The model under review builds one solid part; all positions refer to its coordinate system, in mm. A direction names the side the tool comes from. Coordinates: 2 decimals unless noted, no trailing zeros. Write each loop counter-clockwise with the first axis right and the second up, starting at its lowest first coordinate (ties: lowest second). Pieces come first, ordered by that corner, then holes.
```python
from build123d import *

# Parameters (mm, degrees)
SKETCH2_R           = 1.3
CUT_EXTRUDE1_DEPTH  = 7
SKETCH4_R           = 4.75
CUT_EXTRUDE2_DEPTH  = 82.929848041
FILLET1_R           = 15
FILLET2_R           = 4
SKETCH5_R           = 7
BOSS_EXTRUDE1_DEPTH = 5
CHAMFER1_SIZE       = 1


with BuildPart() as part:
    # Sketch1 → Revolve1 (revolve)
    with BuildSketch(Plane.XY, mode=Mode.PRIVATE) as revolve1_sk:
        Polygon((0, -40), (0, 40), (-12.5, 40), (-12.5, 37), (-8, 28), (-8, -28), (-12.5, -37), (-12.5, -40), align=None)
    revolve(revolve1_sk.sketch.rotate(Axis((0, -40, 0), (0, 1, 0)), 270), axis=Axis((0, -40, 0), (0, 1, 0)))

    # Sketch2 → Cut-Extrude1 (cut)
    with BuildSketch(Plane(origin=(0, 40, 0), x_dir=(1, 0, 0), z_dir=(0, 1, 0))):
        with Locations(Location((-6, 6, 0), (0, 0, 270))):
            Circle(SKETCH2_R)
        with Locations(Location((6, 6, 0), (0, 0, 270))):
            Circle(SKETCH2_R)
        with Locations(Location((-6, -6, 0), (0, 0, 270))):
            Circle(SKETCH2_R)
        with Locations(Location((6, -6, 0), (0, 0, 270))):
            Circle(SKETCH2_R)
    cut_extrude1 = extrude(amount=-CUT_EXTRUDE1_DEPTH, mode=Mode.SUBTRACT)

    # Mirror1: Cut-Extrude1 across plane
    add(cut_extrude1.mirror(Plane.ZX), mode=Mode.SUBTRACT)

    # Sketch3 → Cut-Revolve1 (revolve, cut)
    with BuildSketch(Plane(origin=(0, 0, 0), x_dir=(0, 0, -1), z_dir=(1, 0, 0))):
        Polygon((-5, 31.7), (0, 36.7), (0, -36.7), (-5, -31.7), align=None)
    revolve(axis=Axis((0, 36.7, 0), (0, -1, 0)), mode=Mode.SUBTRACT)

    # Sketch4 → Cut-Extrude2 (cut, through all)
    with BuildSketch(Plane(origin=(0, 40, 0), x_dir=(1, 0, 0), z_dir=(0, 1, 0))):
        with Locations(Location((0, 0, 0), (0, 0, 270))):
            Circle(SKETCH4_R)
    extrude(amount=-CUT_EXTRUDE2_DEPTH, mode=Mode.SUBTRACT)

    # Fillet1
    fillet1_edges = [part.edges().sort_by_distance(p)[0] for p in [
        (0, -28, 8),
        (0, 28, 8),
    ]]
    fillet(fillet1_edges, radius=FILLET1_R)

    # Fillet2
    # the kernel refuses this fillet: 4 mm, written as the material it adds along each edge
    with BuildSketch(Plane(origin=(0, 31.7, 0), x_dir=(0, 0, 1), z_dir=(1, 0, 0))) as fillet2_piece_1:
        with BuildLine():
            CenterArc((1, 1.141941091), FILLET2_R, 339.635865194, 20.364134806)
            Line((5, 1.141941091), (5.08, 1.141941091))
            Line((5.08, 1.141941091), (5.08, 0))
            Line((5.08, 0), (5.056568542, -0.056568542))
            ThreePointArc((5.056568542, -0.056568542), (4.931568542, -0.181568542), (4.825, -0.277838822))
            Line((4.825, -0.277838822), (4.75, -0.25))
        make_face()
    revolve(axis=Axis((0, 31.7, 0), (0, -1, 0)))
    with BuildSketch(Plane(origin=(0, -31.7, 0), x_dir=(0, 0, 1), z_dir=(1, 0, 0))) as fillet2_piece_2:
        with BuildLine():
            CenterArc((1, -1.141941091), FILLET2_R, 0, 20.364134806)
            Line((4.75, 0.25), (4.825, 0.277838822))
            ThreePointArc((4.825, 0.277838822), (4.931568542, 0.181568542), (5.056568542, 0.056568542))
            Line((5.056568542, 0.056568542), (5.08, 0))
            Line((5.08, 0), (5.08, -1.141941091))
            Line((5.08, -1.141941091), (5, -1.141941091))
        make_face()
    revolve(axis=Axis((0, -31.7, 0), (0, -1, 0)))

    # Sketch5 → Boss-Extrude1 (add, symmetric)
    with BuildSketch(Plane(origin=(0, 0, 0), x_dir=(1, 0, 0), z_dir=(0, 1, 0))):
        Polygon((4.618802154, 8), (-4.618802154, 8), (-9.237604307, 0), (-4.618802154, -8), (4.618802154, -8), (9.237604307, 0), align=None)
        Circle(SKETCH5_R, mode=Mode.SUBTRACT)
    extrude(amount=BOSS_EXTRUDE1_DEPTH, both=True)

    # Sketch6 → Cut-Revolve2 (revolve, cut)
    with BuildSketch(Plane.XY, mode=Mode.PRIVATE) as cut_revolve2_sk:
        Polygon((-8, 5), (-9.237604307, 3.762395693), (-9.237604307, 5), align=None)
    cut_revolve2 = revolve(cut_revolve2_sk.sketch.rotate(Axis((0, -40, 0), (0, -1, 0)), 270), axis=Axis((0, -40, 0), (0, -1, 0)), mode=Mode.SUBTRACT)

    # Mirror2: Cut-Revolve2 across plane
    add(cut_revolve2.mirror(Plane.ZX), mode=Mode.SUBTRACT)

    # Chamfer1
    chamfer1_edges = [part.edges().sort_by_distance(p)[0] for p in [
        (0, -40, -4.75),
        (0, 40, -4.75),
    ]]
    chamfer(chamfer1_edges, length=CHAMFER1_SIZE)


solid = part.part
```
Item 1: To check wall thickness, follow line 1 along X through (y, z) = (36.5, 6); line 2 along X through (y, z) = (-35.25, 6); line 3 along X through (y, z) = (-14, 0). State the ranges of each line that lie inside material, in increasing order.
Solved:
line 1: x = -10.68 to -7.3, -4.7 to 4.7, 7.3 to 10.68
line 2: x = -9.96 to -7.3, -4.7 to 4.7, 7.3 to 9.96
line 3: x = -8 to -5, 5 to 8
Item 2: Mouldability with a two-part tool opening along Z and no side actions: class faces 4 (the face through (3.06, 14.59, -7.39)), 5 (the face through (6, 33, 6)), 6 (the face through (4.168, 4.699, 7.179)) as pulls with the +Z half, pulls with the -Z half, needs draft (parallel to the pull), parting line crosses it, or undercut.
Solved:
face 4: parting line crosses it
face 5: undercut
face 6: pulls with the +Z half
Item 3: Machinability: for faces 1 (the face through (4.847, 36.549, 6.6)), 2 (the face through (-4.13, -4.7, 7.2)), 3 (the face through (8.3, 4.7, 0)), which of the approach directions +Z, -Z, +X, -X, +Y, -Y give a long, thin tool a straight path to every point of the face, cutting with its end or side? Answer none if there is none.
Solved:
face 1: +Y
face 2: +Z, -X
face 3: +X
Item 4: For pin 1 (3 mm diameter, centred on x = 6, z = -6, fed in from -Y); pin 2 (1.5 mm diameter, centred on x = 1, y = -14.5, fed in from +Z); pin 3 (1.5 mm diameter, centred on y = -8.5, z = -0.5, fed in from +X); pin 4 (2 mm diameter, centred on y = -13, z = -3, fed in from -X), all flat-tipped, find the tip position at first contact; note any pin that passes through.
Solved:
pin 1: stops at y = -40
pin 2: stops at z = 8
pin 3: stops at x = 8
pin 4: stops at x = -7.75
Item 5: Take a section at A-A, the plane y = -7. Write out the cut boundary in (x, z), plus the area to 3 significant figures.
Solved:
outline: circle Ø16 at (0, 0); hole circle Ø10 at (0, 0)
area: 123 mm2
